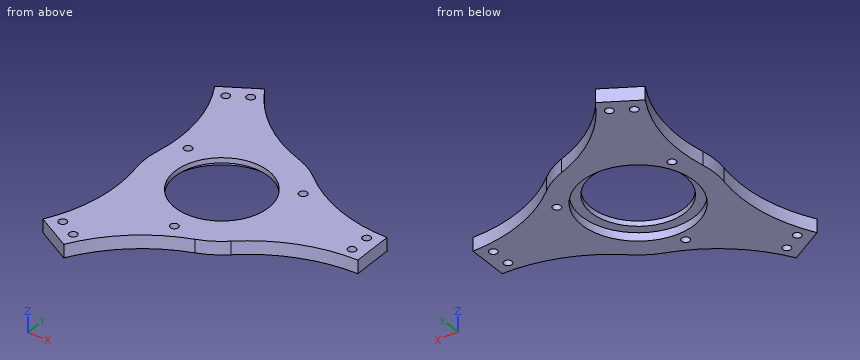
Autodesk Inventor part; units mm, degrees
ref_plane "YZ Plane" through (0, 0, 0) normal (1, 0, 0) x (0, 1, 0)
ref_plane "XZ Plane" through (0, 0, 0) normal (0, 1, 0) x (-1, 0, 0)
ref_plane "XY Plane" through (0, 0, 0) normal (0, 0, 1) x (1, 0, 0)
sketch "Sketch1" plane through (0, 0, 0) normal (0, 0, 1) x (1, 0, 0)
  circle A0 centre (0, 0) radius 55.075
  circle A1 centre (0, 0) radius 75.075
  circle A2 centre (0, -65.075) radius 4
  circle A3 centre (-56.3566, 32.5375) radius 4
  circle A4 centre (56.3566, 32.5375) radius 4
  line L0 (0, -65.075) -> (-56.3566, 32.5375) construction
  line L1 (-56.3566, 32.5375) -> (56.3566, 32.5375) construction
  line L2 (0, -65.075) -> (56.3566, 32.5375) construction
  line L3 (0, -61.075) -> (0, -55.075) construction
  line L4 (-52.8925, 30.5375) -> (-47.6963, 27.5375) construction
  line L5 (47.6963, 27.5375) -> (52.8925, 30.5375) construction
  dimension "d4" = 8
  dimension "d0" = 110.15
  dimension "d1" = 20
  dimension "d6" = 6
extrude "Extrusion1" add sketch "Sketch1" along normal blind 8
sketch "Sketch2" plane through (0, 0, 8) normal (0, 0, 1) x (1, 0, 0)
  circle A0 centre (0, 0) radius 55.075
  circle A1 centre (0, 0) radius 45.75
  circle A2 centre (0, 0) radius 75.075
  circle A3 centre (56.3566, 32.5375) radius 4
  circle A4 centre (-56.3566, 32.5375) radius 4
  circle A5 centre (0, -65.075) radius 4
  circle A6 centre (0, 0) radius 55.075
  dimension "d7" = 91.5
extrude "Extrusion2" add sketch "Sketch2" along normal blind 5 contours A0 | A2
sketch "Sketch3" plane through (0, 0, 13) normal (0, 0, 1) x (1, 0, 0)
  circle A0 centre (0, 0) radius 75.075
  line L0 (72.362, 20) -> (147.404, 20)
  line L1 (147.404, 20) -> (147.404, -20)
  line L2 (147.404, -20) -> (72.362, -20)
  circle A1 centre (0, 0) radius 75.075
  line L3 (-18.8605, -72.6673) -> (-56.3815, -137.6556)
  line L4 (-56.3815, -137.6556) -> (-91.0225, -117.6556)
  line L5 (-91.0225, -117.6556) -> (-53.5015, -52.6673)
  line L6 (-18.8605, 72.6673) -> (-56.3815, 137.6556)
  line L7 (-56.3815, 137.6556) -> (-91.0225, 117.6556)
  line L8 (-91.0225, 117.6556) -> (-53.5015, 52.6673)
  line L9 (147.404, 0) -> (-73.702, 127.6556) construction
  line L10 (-73.702, -127.6556) -> (-73.702, 127.6556) construction
  line L11 (147.404, 0) -> (-73.702, -127.6556) construction
  arc A2 (49.2286, 56.6816) -> (147.404, 20) centre (147.404, 169.7201) ccw
  arc A3 (147.404, -20) -> (49.2286, -56.6816) centre (147.404, -169.7201) ccw
  arc A4 (24.4734, -70.974) -> (-56.3815, -137.6556) centre (73.28, -212.5156) ccw
  arc A5 (-91.0225, -117.6556) -> (-73.702, -14.2925) centre (-220.6839, -42.7955) ccw
  arc A6 (-73.702, 14.2925) -> (-91.0225, 117.6556) centre (-220.6839, 42.7955) ccw
  arc A7 (-56.3815, 137.6556) -> (24.4734, 70.974) centre (73.28, 212.5156) ccw
  point P0 (24.4734, 70.974)
  point P1 (24.4734, -70.974)
  point P2 (-73.702, -14.2925)
  point P3 (49.2286, 56.6816)
  point P4 (49.2286, -56.6816)
  dimension "d10" = 40
extrude "Extrusion3" add sketch "Sketch3" against normal up to surface (13 mm away) contours A0 L0 L1 L2 | A0 A2 L0 | L2 A3 A0 | A0 L6 A7 | A4 L3 A0 | A0 L8 L7 L6 | L3 L4 L5 A0 | A0 A6 L8 | L5 A5 A0
sketch "Sketch4" plane through (0, 0, 0) normal (0, 0, -1) x (-1, 0, 0)
  circle A0 centre (0, 0) radius 135 construction
  circle A1 centre (75.9748, 111.5922) radius 4
  circle A2 centre (58.6543, 121.5922) radius 4
  line L0 (58.6543, 121.5922) -> (56.3815, 137.6556) construction
  line L1 (75.9748, 111.5922) -> (91.0225, 117.6556) construction
  circle A3 centre (-134.6291, -10) radius 4
  circle A4 centre (-134.6291, 10) radius 4
  circle A5 centre (75.9748, -111.5922) radius 4
  circle A6 centre (58.6543, -121.5922) radius 4
  dimension "d13" = 8
  dimension "d14" = 270
  dimension "d15" = 20
  dimension "d18" = 360
extrude "Extrusion4" cut sketch "Sketch4" against normal blind 20
equation "\"d2\" = d4"
properties part number "Tractor_Mobile"
Work out the finished part from the listing and answer in its coordinate system (mm). Coordinates: 2 decimals unless noted, no trailing zeros. Order: outer loops, then holes, each group sorted by start corner. A loop starts at its lowest first (then second) coordinate and runs counter-clockwise, first axis right, second up. Notation, with made-up numbers: (6, 33) - (32, 33) arc R16 cw to (32, 53) - close; hole circle Ø11 at (26, 79.5). An arc over 180 degrees is marked (long way). Put each result on its own line as item: value. Start each with the question number.
1) Flat-ended cylindrical pins translate along their axes: pin 1 (10.5 mm diameter, centred on x = -75.97, y = -111.59, fed in from -Z); pin 2 (6 mm diameter, centred on x = 18.5, z = 8.5, fed in from +Y); pin 3 (6 mm diameter, centred on y = -85, z = 5.5, fed in from -X). Find the tip coordinate at first contact, or state that the pin passes through.
2) Find section D-D (x = 30). Give the vertices of the cut face in (y, z).
3) Find section B-B (x = 0). Give the vertices of the cut face in (y, z) (3 decimals).
4) Find section A-A (y = 0). Give the vertices of the cut face in (x, z) (3 decimals).
5) Find section C-C (z = 2.75). State how many separate pieces and enclosed holes the cut face has, plus the area to 3 significant figures.
6) Find the intervals of material crossed by line 1 (X direction, y = -9, z = 1.25); line 2 (Y direction, x = -2.5, z = 0.75); line 3 (Y direction, x = -58, z = 9.25), in increasing order. Write a range as from..to.
Results list:
1. pin 1: stops at z = 0
1. pin 2: stops at y = 74.39
1. pin 3: stops at x = -77.95
2. outline: (-68.82, 0) - (-46.19, 0) - (-46.19, 8) - (-34.54, 8) - (-34.54, 13) - (-68.82, 13) - close; (34.54, 8) - (46.19, 8) - (46.19, 0) - (68.82, 0) - (68.82, 13) - (34.54, 13) - close
3. outline: (-81.955, 0) - (-69.075, 0) - (-69.075, 13) - (-81.955, 13) - close; (-61.075, 0) - (-55.075, 0) - (-55.075, 8) - (-45.75, 8) - (-45.75, 13) - (-61.075, 13) - close; (45.75, 8) - (55.075, 8) - (55.075, 0) - (81.955, 0) - (81.955, 13) - (45.75, 13) - close
4. outline: (-75.075, 0) - (-55.075, 0) - (-55.075, 8) - (-45.75, 8) - (-45.75, 13) - (-75.075, 13) - close; (45.75, 8) - (55.075, 8) - (55.075, 0) - (147.404, 0) - (147.404, 13) - (45.75, 13) - close
5. separate pieces: 1
5. enclosed holes: 10
5. area: 20,200 mm^2
6. line 1: x = -74.53..-54.33, 54.33..130.76, 138.5..147.4
6. line 2: y = -83.39..-68.2, -61.95..-55.02, 55.02..83.39
6. line 3: y = -136.72..-125.54, -117.65..28.89, 36.18..117.65, 125.54..136.72
